from build123d import *

# Parameters (mm, degrees)
F_5_16_CLEARANCE_HOLE1_D   = 8.4328
CIRPATTERN1_COUNT          = 12
F_1_2_0_4_DIAMETER_HOLE1_D = 10.16
CIRPATTERN2_COUNT          = 6
CUT_EXTRUDE1_DEPTH         = 25.4
CUT_EXTRUDE2_DEPTH         = 112.584919067
CUT_EXTRUDE2_DEPTH_BACK    = 107.174719067
SKETCH36_R                 = 9.7155
SKETCH36_R_2               = 6.6675
CUT_EXTRUDE3_DEPTH         = 2.54


with BuildPart() as part:
    # Sketch1 → Revolve1 (revolve)
    with BuildSketch(Plane.XY):
        Polygon((-54.356, 0), (-88.9, 0), (-88.9, 44.45), (0, 44.45), (0, 19.05), (-14.2875, 19.05), (-14.2875, 6.35), (-20.6375, 6.35), (-20.6375, 0), (-50.8, 0), (-50.8, 2.54), (-54.356, 2.54), align=None)
    revolve(axis=Axis((0, 0, 0), (0, 1, 0)))

    # 5_16 Clearance Hole1 (through all)
    with Locations(Plane(origin=(0, 44.45, 0), x_dir=(1, 0, 0), z_dir=(0, 1, 0))):
        with Locations((-73.603547963, -19.722011237)):
            f_5_16_clearance_hole1 = Hole(F_5_16_CLEARANCE_HOLE1_D / 2)

    # CirPattern1: 5_16 Clearance Hole1 ×12 about axis
    cirpattern1_axis = Axis((0, 0, 0), (0, 1, 0))
    for i in range(1, CIRPATTERN1_COUNT):
        add(f_5_16_clearance_hole1.rotate(cirpattern1_axis, i * 360 / CIRPATTERN1_COUNT), mode=Mode.SUBTRACT)

    # Sketch19 → 3_8 NPT Tapped Hole1 (revolve, cut)
    with BuildSketch(Plane(origin=(10.682756087, 44.45, 39.86858848), x_dir=(0, 0, 1), z_dir=(1, 0, 0))):
        Polygon((0, 0), (0, 44.45), (7.1374, 44.45), (7.1374, 10.414), (7.653732494, 10.414), (7.9655416, 0), align=None)
    f_3_8_npt_tapped_hole1 = revolve(axis=Axis((10.682756087, 50.8, 39.86858848), (0, -1, 0)), mode=Mode.SUBTRACT)

    # Mirror1: 3_8 NPT Tapped Hole1 across plane
    add(f_3_8_npt_tapped_hole1.mirror(Plane(origin=(0, 0, 0), x_dir=(0.965925826, 0, -0.258819045), z_dir=(-0.258819045, 0, -0.965925826))), mode=Mode.SUBTRACT)

    # 1_2 _0.4_ Diameter Hole1 (through all)
    with Locations(Plane(origin=(0, 44.45, 0), x_dir=(1, 0, 0), z_dir=(0, 1, 0))):
        with Locations((30.668144985, 8.217504682)):
            Hole(F_1_2_0_4_DIAMETER_HOLE1_D / 2)

    # Sketch30 → Tap Drill for 1_4-28 Tap1 (revolve, cut)
    with BuildSketch(Plane(origin=(55.202660972, 44.45, -14.791508428), x_dir=(0, 0, 1), z_dir=(1, 0, 0))):
        Polygon((0, 0), (0, 17.500388061), (2.7051, 15.875), (2.7051, 0), align=None)
    tap_drill_for_1_4_28_tap1 = revolve(axis=Axis((55.202660972, 50.8, -14.791508428), (0, -1, 0)), mode=Mode.SUBTRACT)

    # CirPattern2: Tap Drill for 1_4-28 Tap1 ×6 about axis
    cirpattern2_axis = Axis((30.668144985, 0, -8.217504682), (0, 1, 0))
    for i in range(1, CIRPATTERN2_COUNT):
        add(tap_drill_for_1_4_28_tap1.rotate(cirpattern2_axis, i * 360 / CIRPATTERN2_COUNT), mode=Mode.SUBTRACT)

    # Sketch31 → Cut-Extrude1 (cut)
    with BuildSketch(Plane(origin=(0, 44.45, 0), x_dir=(1, 0, 0), z_dir=(0, 1, 0))):
        with BuildLine():
            Line((0, -63.5), (6.737403156, -88.644330889))
            ThreePointArc((6.737403156, -88.644330889), (-85.870805957, -23.00901311), (-38.487403156, 80.136944029))
            Line((-38.487403156, 80.136944029), (-31.75, 54.99261314))
            ThreePointArc((-31.75, 54.99261314), (-61.336289969, -16.435009364), (0, -63.5))
        make_face()
    extrude(amount=-CUT_EXTRUDE1_DEPTH, mode=Mode.SUBTRACT)

    # Sketch33 → Cut-Extrude2 (cut, two sides)
    with BuildSketch(Plane(origin=(0.700131399, 0, 2.612925953), x_dir=(-0.965925826, 0, 0.258819045), z_dir=(-0.258819045, 0, -0.965925826))) as cut_extrude2_sk:
        Polygon((16.435009364, 44.45), (41.835009364, 19.05), (63.5, 19.05), (63.5, 44.45), align=None)
    extrude(amount=CUT_EXTRUDE2_DEPTH, mode=Mode.SUBTRACT)
    extrude(cut_extrude2_sk.sketch, amount=-CUT_EXTRUDE2_DEPTH_BACK, mode=Mode.SUBTRACT)

    # Sketch35 → 1_2 NPT Tapped Hole1 (revolve, cut)
    with BuildSketch(Plane(origin=(-24.549261314, 35.469743879, 6.577954744), x_dir=(-0.365367827, -0.547722558, 0.752666162), z_dir=(0.632455532, 0.447213595, 0.632455532))):
        Polygon((0, 0), (0, 40.289543693), (8.9281, 34.925), (8.9281, 13.462), (9.479726792, 13.462), (9.8827971, 0), align=None)
    revolve(axis=Axis((-28.886391971, 39.959871939, 7.740085401), (0.683012702, -0.707106781, -0.183012702)), mode=Mode.SUBTRACT)

    # Sketch36 → Cut-Extrude3 (cut)
    with BuildSketch(Plane.XZ):
        with Locations((30.668144985, -8.217504682)):
            Circle(SKETCH36_R)
        with Locations((30.668144985, -8.217504682)):
            Circle(SKETCH36_R_2, mode=Mode.SUBTRACT)
    extrude(amount=-CUT_EXTRUDE3_DEPTH, mode=Mode.SUBTRACT)


solid = part.part
Check sheet for the modelled part. Datum: model origin and axes. Units: mm. A direction names the side the tool comes from. Coordinates: 2 decimals unless noted, no trailing zeros. Write each loop counter-clockwise with the first axis right and the second up, starting at its lowest first coordinate (ties: lowest second). Pieces come first, ordered by that corner, then holes. Notation, with made-up numbers: M -19.75,31.5 L 19.25,31.5 A13 ccw 19.25,54.5 Z; hole C 37.5,53 d2. An arc over 180 degrees is marked long. Answer as CSV lines item,"result".
Q1. Cross-section at A-A (x = 29.5). Record the boundary of the cut face in (y, z).
Check result:
outline,"M 0,-83.86 L 44.45,-83.86 L 44.45,-13.16 L 0,-13.16 L 0,-14.78 L 2.54,-14.78 L 2.54,-17.86 L 0,-17.86 L 0,-41.36 L 2.54,-41.36 L 2.54,-45.65 L 0,-45.65 Z; M 0,-3.27 L 44.45,-3.27 L 44.45,83.86 L 0,83.86 L 0,45.65 L 2.54,45.65 L 2.54,41.36 L 0,41.36 L 0,1.43 L 2.54,1.43 L 2.54,-1.65 L 0,-1.65 Z"
Q2. Set-up check for faces 5 (the face through (-12.376, 39.316, -32.243)), 6 (the face through (28, 2.54, -15)), 7 (the face through (-35.166, 31.928, -67.741)), 8 (the face through (26, 44.45, -19)), 9 (the face through (-77.784, 9.392, -20.271)): record each of +Z, -Z, +X, -X, +Y, -Y from which the full face is reachable in a straight line by a thin tool's end or side.
Check result:
face 5,"+Y"
face 6,"-Y"
face 7,"-X, +Y"
face 8,"+Z, -Z, +X, -X, +Y"
face 9,"+Y, -Y"
Q3. Material ranges on probe 1 along Z at (x, y) = (0, 0.85); probe 2 along Z at (x, y) = (71, 25.5); probe 3 along X at (y, z) = (39.5, 21), recorded low to high. Write a range as from..to.
Check result:
probe 1,"-88.9..-54.36, -50.8..-20.64, 20.64..50.8, 54.36..88.9"
probe 2,"-53.5..-23.04, -16.41..16.41, 23.04..53.5"
probe 3,"-16.51..69.59, 77.62..86.38"
Q4. Mould release check, pull along X, two halves, no side actions. Record for faces 1 (the face through (-8.25, 26.28, 62.96)), 2 (the face through (-41, 0, -38)), 3 (the face through (-49.99, 9.39, -55.5)), 4 (the face through (15.44, 39.32, 33.67)): released by +X, released by -X, zero draft, split by the parting line, or undercut.
Check result:
face 1,"released by -X"
face 2,"zero draft"
face 3,"undercut"
face 4,"undercut"
Q5. Cross-section at B-B (y = 39). Count the separate pieces of the cut face and the enclosed holes in it, then the cut area to 3 significant figures.
Check result:
separate pieces,"1"
enclosed holes,"16"
area,"14,900 mm^2"
Q6. Go/stop test with flat-tipped pins: pin 1 (10 mm diameter, centred on y = 21.5, z = -9, fed in from +X); pin 2 (6 mm diameter, centred on x = -69, y = 13.5, fed in from +Z); pin 3 (5 mm diameter, centred on x = 24.09, z = 16.32, fed in from +Y). Record where each tip stops, or that it passes through.
Check result:
pin 1,"x = 88.81"
pin 2,"z = 59.56"
pin 3,"y = 28.45"
